```python
from build123d import *

# Parameters (mm, degrees)
SKETCH1_R           = 1.35
BOSS_EXTRUDE1_DEPTH = 6
SKETCH2_R           = 2.5
SKETCH2_R_2         = 1.35
CUT_EXTRUDE1_DEPTH  = 3
SKETCH3_R           = 3.175
SKETCH3_R_2         = 1.35
BOSS_EXTRUDE2_DEPTH = 3
CUT_EXTRUDE2_START  = -3
CUT_EXTRUDE2_DEPTH  = 3
SKETCH7_R           = 5.6
CUT_EXTRUDE3_DEPTH  = 10
CUT_EXTRUDE4_START  = -3.5
SKETCH8_R           = 8
SKETCH8_R_2         = 5.6
CUT_EXTRUDE4_DEPTH  = 3.5
SKETCH9_W           = 5
SKETCH9_H           = 7
CUT_EXTRUDE5_DEPTH  = 92.268613627


with BuildPart() as part:
    # Sketch1 → Boss-Extrude1 (new body)
    with BuildSketch(Plane(origin=(0, 0, 0), x_dir=(1, 0, 0), z_dir=(0, 1, 0))):
        with BuildLine():
            Line((-52.2, 66.182473763), (52.2, 66.182473763))
            ThreePointArc((52.2, 66.182473763), (59.271067812, 63.253541574), (62.2, 56.182473763))
            Line((62.2, 56.182473763), (62.2, -46.121814954))
            ThreePointArc((62.2, -46.121814954), (59.271067812, -53.192882766), (52.2, -56.121814954))
            Line((52.2, -56.121814954), (-52.2, -56.121814954))
            ThreePointArc((-52.2, -56.121814954), (-59.271067812, -53.192882766), (-62.2, -46.121814954))
            Line((-62.2, -46.121814954), (-62.2, 56.182473763))
            ThreePointArc((-62.2, 56.182473763), (-59.271067812, 63.253541574), (-52.2, 66.182473763))
        make_face()
        with Locations(Location((-48, -44.121814954, 0), (0, 0, 270))):
            Circle(SKETCH1_R, mode=Mode.SUBTRACT)
        with Locations(Location((-52.2, 47.982473763, 0), (0, 0, 270))):
            Circle(SKETCH1_R, mode=Mode.SUBTRACT)
        with Locations(Location((52.2, 47.982473763, 0), (0, 0, 270))):
            Circle(SKETCH1_R, mode=Mode.SUBTRACT)
        with Locations(Location((48, -44.121814954, 0), (0, 0, 270))):
            Circle(SKETCH1_R, mode=Mode.SUBTRACT)
    extrude(amount=BOSS_EXTRUDE1_DEPTH)

    # Sketch2 → Cut-Extrude1 (cut)
    # profile 1 of 4: a face of its own
    with BuildSketch(Plane.XZ):
        with Locations(Location((-48, 44.121814954, 0), (0, 0, 270))):
            Circle(SKETCH2_R)
        with Locations(Location((-48, 44.121814954, 0), (0, 0, 270))):
            Circle(SKETCH2_R_2, mode=Mode.SUBTRACT)
    # profile 2 of 4: a face of its own
    with BuildSketch(Plane.XZ):
        with Locations(Location((-52.2, -47.982473763, 0), (0, 0, 270))):
            Circle(SKETCH2_R)
        with Locations(Location((-52.2, -47.982473763, 0), (0, 0, 270))):
            Circle(SKETCH2_R_2, mode=Mode.SUBTRACT)
    # profile 3 of 4: a face of its own
    with BuildSketch(Plane.XZ):
        with Locations(Location((52.2, -47.982473763, 0), (0, 0, 270))):
            Circle(SKETCH2_R)
        with Locations(Location((52.2, -47.982473763, 0), (0, 0, 270))):
            Circle(SKETCH2_R_2, mode=Mode.SUBTRACT)
    # profile 4 of 4: a face of its own
    with BuildSketch(Plane.XZ):
        with Locations(Location((48, 44.121814954, 0), (0, 0, 270))):
            Circle(SKETCH2_R)
        with Locations(Location((48, 44.121814954, 0), (0, 0, 270))):
            Circle(SKETCH2_R_2, mode=Mode.SUBTRACT)
    extrude(amount=-CUT_EXTRUDE1_DEPTH, mode=Mode.SUBTRACT)

    # Sketch3 → Boss-Extrude2 (add)
    # profile 1 of 4: a face of its own
    with BuildSketch(Plane(origin=(0, 6, 0), x_dir=(1, 0, 0), z_dir=(0, 1, 0))):
        with Locations(Location((-52.2, 47.982473763, 0), (0, 0, 270))):
            Circle(SKETCH3_R)
        with Locations(Location((-52.2, 47.982473763, 0), (0, 0, 90))):
            Circle(SKETCH3_R_2, mode=Mode.SUBTRACT)
    # profile 2 of 4: a face of its own
    with BuildSketch(Plane(origin=(0, 6, 0), x_dir=(1, 0, 0), z_dir=(0, 1, 0))):
        with Locations(Location((52.2, 47.982473763, 0), (0, 0, 270))):
            Circle(SKETCH3_R)
        with Locations(Location((52.2, 47.982473763, 0), (0, 0, 90))):
            Circle(SKETCH3_R_2, mode=Mode.SUBTRACT)
    # profile 3 of 4: a face of its own
    with BuildSketch(Plane(origin=(0, 6, 0), x_dir=(1, 0, 0), z_dir=(0, 1, 0))):
        with Locations(Location((48, -44.121814954, 0), (0, 0, 270))):
            Circle(SKETCH3_R)
        with Locations(Location((48, -44.121814954, 0), (0, 0, 90))):
            Circle(SKETCH3_R_2, mode=Mode.SUBTRACT)
    # profile 4 of 4: a face of its own
    with BuildSketch(Plane(origin=(0, 6, 0), x_dir=(1, 0, 0), z_dir=(0, 1, 0))):
        with Locations(Location((-48, -44.121814954, 0), (0, 0, 270))):
            Circle(SKETCH3_R)
        with Locations(Location((-48, -44.121814954, 0), (0, 0, 90))):
            Circle(SKETCH3_R_2, mode=Mode.SUBTRACT)
    extrude(amount=BOSS_EXTRUDE2_DEPTH)

    # Sketch4 → Cut-Extrude2 (cut)
    with BuildSketch(Plane(origin=(0, 6, 0), x_dir=(1, 0, 0), z_dir=(0, 1, 0)).offset(CUT_EXTRUDE2_START)):
        with BuildLine():
            Line((52.2, 66.182473763), (-52.2, 66.182473763))
            ThreePointArc((-52.2, 66.182473763), (-59.271067812, 63.253541574), (-62.2, 56.182473763))
            Line((-62.2, 56.182473763), (-62.2, -46.121814954))
            ThreePointArc((-62.2, -46.121814954), (-59.271067812, -53.192882766), (-52.2, -56.121814954))
            Line((-52.2, -56.121814954), (52.2, -56.121814954))
            ThreePointArc((52.2, -56.121814954), (59.271067812, -53.192882766), (62.2, -46.121814954))
            Line((62.2, -46.121814954), (62.2, 56.182473763))
            ThreePointArc((62.2, 56.182473763), (59.271067812, 63.253541574), (52.2, 66.182473763))
        make_face()
        with BuildLine():
            Line((-60.6, 56.182473763), (-60.6, -46.121814954))
            ThreePointArc((-60.6, -46.121814954), (-58.139696962, -52.061511916), (-52.2, -54.521814954))
            Line((-52.2, -54.521814954), (52.2, -54.521814954))
            ThreePointArc((52.2, -54.521814954), (58.139696962, -52.061511916), (60.6, -46.121814954))
            Line((60.6, -46.121814954), (60.6, 56.182473763))
            ThreePointArc((60.6, 56.182473763), (58.139696962, 62.122170725), (52.2, 64.582473763))
            Line((52.2, 64.582473763), (-52.2, 64.582473763))
            ThreePointArc((-52.2, 64.582473763), (-58.139696962, 62.122170725), (-60.6, 56.182473763))
        make_face(mode=Mode.SUBTRACT)
    extrude(amount=CUT_EXTRUDE2_DEPTH, mode=Mode.SUBTRACT)

    # Sketch7 → Cut-Extrude3 (cut)
    with BuildSketch(Plane(origin=(0, 6, 0), x_dir=(1, 0, 0), z_dir=(0, 1, 0))):
        with Locations(Location((-32.2, 55.982473763, 0), (0, 0, 270))):
            Circle(SKETCH7_R)
    extrude(amount=-CUT_EXTRUDE3_DEPTH, mode=Mode.SUBTRACT)

    # Sketch8 → Cut-Extrude4 (cut)
    with BuildSketch(Plane.XZ.offset(CUT_EXTRUDE4_START)):
        with Locations(Location((-32.2, -55.982473763, 0), (0, 0, 270))):
            Circle(SKETCH8_R)
        with Locations(Location((-32.2, -55.982473763, 0), (0, 0, 90))):
            Circle(SKETCH8_R_2, mode=Mode.SUBTRACT)
    extrude(amount=CUT_EXTRUDE4_DEPTH, mode=Mode.SUBTRACT)

    # Sketch9 → Cut-Extrude5 (cut, through all)
    with BuildSketch(Plane.XZ):
        with Locations((41.9, 47.621814954)):
            Rectangle(SKETCH9_W, SKETCH9_H)
    extrude(amount=-CUT_EXTRUDE5_DEPTH, mode=Mode.SUBTRACT)


solid = part.part
```
CAD build for the part. Positions are in the model's coordinates, mm. A direction names the side the tool comes from. Coordinates: 2 decimals unless noted, no trailing zeros. Order: outer loops, then holes, each group sorted by start corner. A loop starts at its lowest first (then second) coordinate and runs counter-clockwise, first axis right, second up. Notation, with made-up numbers: M 9.5,17.25 L 63.5,17.25 A17 cw 63.5,24.25 Z; hole C 74.5,-3.75 d9. An arc over 180 degrees is marked long. Write each question's results on one line, items separated by ' | '. Start each with the question number.
Q1. Cut at D-D (x = -8). List the corners of the cut face in (y, z).
Q2. Pull direction X, two halves, no side cores. Call faces 5 (the cylindrical face through (-58.07, 4.48, -62.19)), 6 (the flat face through (42, 3, 44.122)), 7 (the flat face through (-1, 1, -66.182)): +X half, -X half, draft (parallel to the pull), parting line (faces both ways), or undercut.
Q3. Which spindle directions (+Z, -Z, +X, -X, +Y, -Y) get a long thin tool onto all of the face, cutting with end or side? Do faces 1 (the cylindrical face through (-50.05, 7.48, -50.32)), 2 (the flat face through (42, 3, 51.122)), 3 (the flat face through (-30.3, 3.5, -50.5)), 4 (the flat face through (-60.6, 4, -6)). Say none if no direction does.
Q4. Cut at B-B (x = -32.2). List the corners of the cut face in (y, z).
Q5. Flat gauge pins, fed straight in: P1, Ø6.5, axis at x = -32.2, z = -55.98, coming from the +Y side; P2, Ø1, axis at x = -2.5, z = 6.5, coming from the +Y side; P3, Ø2.5, axis at x = -10.5, y = 5, coming from the +Z side; P4, Ø4, axis at x = 48, z = 44.12, coming from the -Y side. Where does each tip first touch, or does it go through?
Q6. Drill centre lines: probe 1 along X at (y, z) = (4.5, 44); probe 2 along Y at (x, z) = (-15.5, -39); probe 3 along X at (y, z) = (5.5, 31). Where is each one in solid material? Low to high. Write a range as from..to.
Q7. Cut at C-C (z = 20). List the corners of the cut face in (x, y), then the cut area to 3 significant figures.
Q8. Cut at A-A (y = 1.5). List the corners of the cut face in (x, z).
Found:
1) outline: M 0,-66.18 L 3,-66.18 L 3,-64.58 L 6,-64.58 L 6,54.52 L 3,54.52 L 3,56.12 L 0,56.12 Z
2) face 5: -X half | face 6: undercut | face 7: draft
3) face 1: +Y | face 2: +Y, -Y | face 3: -Y | face 4: +Z, -Z, -X, +Y
4) outline: M 0,-66.18 L 3,-66.18 L 3,-64.58 L 6,-64.58 L 6,-61.58 L 3.5,-61.58 L 3.5,-63.98 L 0,-63.98 Z; M 0,-47.98 L 3.5,-47.98 L 3.5,-50.38 L 6,-50.38 L 6,54.52 L 3,54.52 L 3,56.12 L 0,56.12 Z
5) P1: through | P2: y = 6 | P3: z = 54.52 | P4: y = 3
6) probe 1: -60.6..-49.34, -46.66..46.66, 49.34..60.6 | probe 2: 0..6 | probe 3: -60.6..60.6
7) outline: M -62.2,0 L 62.2,0 L 62.2,3 L 60.6,3 L 60.6,6 L -60.6,6 L -60.6,3 L -62.2,3 Z | area: 737 mm²
8) outline: M -62.2,-56.18 A10 ccw -52.2,-66.18 L 52.2,-66.18 A10 ccw 62.2,-56.18 L 62.2,46.12 A10 ccw 52.2,56.12 L -52.2,56.12 A10 ccw -62.2,46.12 Z; hole C -52.2,-47.98 d5; hole C -48,44.12 d5; hole C -32.2,-55.98 d16; hole M 39.4,44.12 L 44.4,44.12 L 44.4,51.12 L 39.4,51.12 Z; hole C 48,44.12 d5; hole C 52.2,-47.98 d5
